The model under review builds one solid part; all positions refer to its coordinate system, in mm. A direction names the side the tool comes from. Round coordinates to 2 decimals unless told otherwise and drop trailing zeros. Write each loop counter-clockwise with the first axis right and the second up, starting at its lowest first coordinate (ties: lowest second). Pieces come first, ordered by that corner, then holes. Notation, with made-up numbers: (11.5, 72.25) -> (40.5, 72.25) arc R26 ccw to (40.5, 102.25) -> close; hole circle Ø8 at (67.25, 77.25). An arc over 180 degrees is marked (long way). Use CSV: the item, a comma, the result in double quotes. Start each with the question number.
1) Take a section at C-C, the plane x = -0.75. Give the boundary of the cut face in (y, z), then the cut area to 3 significant figures.
2) Machinability: for faces 1 (the face through (12.099, -0.178, 12.066)), 2 (the face through (10.49, 0, 0)), 3 (the face through (0, 0, 4.517)), which of the approach directions +Z, -Z, +X, -X, +Y, -Y give a long, thin tool a straight path to every point of the face, cutting with its end or side? Answer none if there is none.
3) Take a section at B-B, the plane z = -6. Give the boundary of the cut face in (x, y), then the cut area to 3 significant figures.
4) Take a section at A-A, the plane z = 11. Give the boundary of the cut face in (x, y), then the cut area to 3 significant figures.
5) For pin 1 Ø2.5 at (x, y) = (0, -3.5) entering from +Z; pin 2 Ø0.8 at (x, z) = (-2.47, 2.47) entering from -Y; pin 3 Ø3.5 at (y, z) = (4.5, -0.5) entering from -X, all flat-tipped, find the tip position at first contact; note any pin that passes through.
6) Take a section at D-D, the plane y = -11. State how many separate pieces and enclosed holes the cut face has, then the cut area to 3 significant figures.
7) Wall thickness on probe 1 along X at (y, z) = (5.5, -8.75); probe 2 along Z at (x, y) = (-4.25, 4.25) (3 decimals); probe 3 along Z at (x, y) = (-6.75, -10.5): over which ranges is each line inside the solid? List them lowest first. Write a range as [from, to].
Autodesk Inventor part; units mm, degrees
ref_plane "YZ Plane" through (0, 0, 0) normal (1, 0, 0) x (0, 1, 0)
ref_plane "XZ Plane" through (0, 0, 0) normal (0, 1, 0) x (-1, 0, 0)
ref_plane "XY Plane" through (0, 0, 0) normal (0, 0, 1) x (1, 0, 0)
sketch "Sketch1" plane through (0, 0, 0) normal (0, 1, 0) x (-1, 0, 0)
  arc A0 (-1.9692, 2.8605) -> (-2.8605, 1.9692) centre (-2.4696, 2.4696) ccw
  line L0 (-2.2319, 1.3405) -> (-2.8605, 1.9692)
  arc A1 (-2.2319, 1.3405) -> (-2.2319, -1.3405) centre (0, 0) ccw
  line L1 (-2.8605, -1.9692) -> (-2.2319, -1.3405)
  arc A2 (-2.8605, -1.9692) -> (-1.9692, -2.8605) centre (-2.4696, -2.4696) ccw
  line L2 (-1.3405, -2.2319) -> (-1.9692, -2.8605)
  arc A3 (-1.3405, -2.2319) -> (1.3405, -2.2319) centre (0, 0) ccw
  line L3 (1.9692, -2.8605) -> (1.3405, -2.2319)
  arc A4 (1.9692, -2.8605) -> (2.8605, -1.9692) centre (2.4696, -2.4696) ccw
  line L4 (2.2319, -1.3405) -> (2.8605, -1.9692)
  arc A5 (2.2319, -1.3405) -> (2.2319, 1.3405) centre (0, 0) ccw
  line L5 (2.8605, 1.9692) -> (2.2319, 1.3405)
  arc A6 (2.8605, 1.9692) -> (1.9692, 2.8605) centre (2.4696, 2.4696) ccw
  line L6 (1.3405, 2.2319) -> (1.9692, 2.8605)
  arc A7 (1.3405, 2.2319) -> (-1.3405, 2.2319) centre (0, 0) ccw
  line L7 (-1.9692, 2.8605) -> (-1.3405, 2.2319)
  arc A8 (-8.7558, 7.1932) -> (-10.4902, 6.4748) centre (-9.4742, 6.4748) ccw
  line L8 (-10.4902, -6.4748) -> (-10.4902, 6.4748)
  arc A9 (-10.4902, -6.4748) -> (-8.7558, -7.1932) centre (-9.4742, -6.4748) ccw
  line L9 (-5.4471, -3.8845) -> (-8.7558, -7.1932)
  arc A10 (-5.4471, -3.8845) -> (-4.5172, -1.6395) centre (-7.6922, -1.6395) ccw
  line L10 (-4.5172, 1.6395) -> (-4.5172, -1.6395)
  arc A11 (-4.5172, 1.6395) -> (-5.4471, 3.8845) centre (-7.6922, 1.6395) ccw
  line L11 (-8.7558, 7.1932) -> (-5.4471, 3.8845)
  arc A12 (3.8845, -5.4471) -> (1.6395, -4.5172) centre (1.6395, -7.6922) ccw
  line L12 (-1.6395, -4.5172) -> (1.6395, -4.5172)
  arc A13 (-1.6395, -4.5172) -> (-3.8845, -5.4471) centre (-1.6395, -7.6922) ccw
  line L13 (-7.1932, -8.7558) -> (-3.8845, -5.4471)
  arc A14 (-7.1932, -8.7558) -> (-6.4748, -10.4902) centre (-6.4748, -9.4742) ccw
  line L14 (6.4748, -10.4902) -> (-6.4748, -10.4902)
  arc A15 (6.4748, -10.4902) -> (7.1932, -8.7558) centre (6.4748, -9.4742) ccw
  line L15 (3.8845, -5.4471) -> (7.1932, -8.7558)
  arc A16 (-12.7002, -10.5921) -> (-10.592, -12.7003) centre (-10.592, -10.5921) ccw
  line L16 (-12.7002, -10.5921) -> (-12.7002, 10.5915)
  arc A17 (-10.592, 12.6997) -> (-12.7002, 10.5915) centre (-10.592, 10.5915) ccw
  line L17 (-10.592, 12.6997) -> (-4.3561, 12.6997)
  arc A18 (-4.3561, 10.4899) -> (-4.3561, 12.6997) centre (-4.3561, 11.5948) ccw
  line L18 (-4.3561, 10.4899) -> (-6.4746, 10.4899)
  arc A19 (-6.4746, 10.4899) -> (-7.193, 8.7555) centre (-6.4746, 9.4739) ccw
  line L19 (-7.193, 8.7555) -> (-3.8847, 5.4472)
  arc A20 (-3.8847, 5.4472) -> (-1.6396, 4.5172) centre (-1.6396, 7.6922) ccw
  line L20 (-1.6396, 4.5172) -> (1.6395, 4.5172)
  arc A21 (1.6395, 4.5172) -> (3.8846, 5.4472) centre (1.6395, 7.6922) ccw
  line L21 (3.8846, 5.4472) -> (7.1929, 8.7555)
  arc A22 (7.1929, 8.7555) -> (6.4745, 10.4899) centre (6.4745, 9.4739) ccw
  line L22 (6.4745, 10.4899) -> (4.3561, 10.4899)
  arc A23 (4.3561, 12.6997) -> (4.3561, 10.4899) centre (4.3561, 11.5948) ccw
  line L23 (4.3561, 12.6997) -> (10.592, 12.6997)
  arc A24 (12.7002, 10.5915) -> (10.592, 12.6997) centre (10.592, 10.5915) ccw
  line L24 (12.7002, 10.5915) -> (12.7002, 4.3561)
  arc A25 (10.4904, 4.3561) -> (12.7002, 4.3561) centre (11.5953, 4.3561) ccw
  line L25 (10.4904, 4.3561) -> (10.4904, 6.475)
  arc A26 (10.4904, 6.475) -> (8.756, 7.1934) centre (9.4744, 6.475) ccw
  line L26 (8.756, 7.1934) -> (5.4472, 3.8846)
  arc A27 (5.4472, 3.8846) -> (4.5172, 1.6395) centre (7.6922, 1.6395) ccw
  line L27 (4.5172, 1.6395) -> (4.5172, -1.6396)
  arc A28 (4.5172, -1.6396) -> (5.4472, -3.8847) centre (7.6922, -1.6396) ccw
  line L28 (5.4472, -3.8847) -> (8.756, -7.1935)
  arc A29 (8.756, -7.1935) -> (10.4904, -6.4751) centre (9.4744, -6.4751) ccw
  line L29 (10.4904, -6.4751) -> (10.4904, -4.3561)
  arc A30 (12.7002, -4.3561) -> (10.4904, -4.3561) centre (11.5953, -4.3561) ccw
  line L30 (12.7002, -4.3561) -> (12.7002, -10.5921)
  arc A31 (10.592, -12.7003) -> (12.7002, -10.5921) centre (10.592, -10.5921) ccw
  line L31 (10.592, -12.7003) -> (-10.592, -12.7003)
  point P0 (0, 0)
  dimension "d23" = 8.183
  dimension "d69" = 1.016
  dimension "d70" = 3.175
  dimension "d86" = 17.2174
  dimension "d87" = 23.1904
  dimension "d88" = 25.4004
  dimension "d89" = 17.2169
  dimension "d90" = 23.1899
  dimension "d92" = 8.1825
  dimension "d93" = 2.2098
  dimension "d96" = 2.2097
extrude "Extrusion1" add sketch "Sketch1" along normal mid plane 25.4
properties part number "1002-S-BLACK-FB" material "6105-T5"
Values found:
1,outline,"(-12.7, -12.7) -> (12.7, -12.7) -> (12.7, -10.49) -> (-12.7, -10.49) -> close; (-12.7, -4.52) -> (12.7, -4.52) -> (12.7, -2.49) -> (-12.7, -2.49) -> close; (-12.7, 2.49) -> (12.7, 2.49) -> (12.7, 4.52) -> (-12.7, 4.52) -> close"
1,area,"159 mm²"
2,face 1,"+Z, +X, +Y, -Y"
2,face 2,"+Y, -Y"
2,face 3,"+Z, +Y, -Y"
3,outline,"(-12.7, -12.7) -> (-10.49, -12.7) -> (-10.49, 12.7) -> (-12.7, 12.7) -> close; (-7.56, -12.7) -> (-4.44, -12.7) -> (-4.44, 12.7) -> (-7.56, 12.7) -> close; (4.44, -12.7) -> (7.56, -12.7) -> (7.56, 12.7) -> (4.44, 12.7) -> close; (10.49, -12.7) -> (12.7, -12.7) -> (12.7, 12.7) -> (10.49, 12.7) -> close"
3,area,"271 mm²"
4,outline,"(-12.66, -12.7) -> (-3.42, -12.7) -> (-3.42, 12.7) -> (-12.66, 12.7) -> close; (3.42, -12.7) -> (12.66, -12.7) -> (12.66, 12.7) -> (3.42, 12.7) -> close"
4,area,"469 mm²"
5,pin 1,"z = 4.52"
5,pin 2,"through"
5,pin 3,"x = -4.58"
6,separate pieces,"1"
6,enclosed holes,"3"
6,area,"310 mm²"
7,probe 1,"[-12.7, -7.19], [7.19, 12.7]"
7,probe 2,"[-12.7, -10.49], [-5.813, 5.813], [10.495, 12.695]"
7,probe 3,"[-12.7, -10.45], [-8.31, -5.19], [5.19, 8.31], [10.45, 12.7]"
